Can you work these out from the model? Positions are in its coordinate system, mm. Round coordinates to 2 decimals unless told otherwise and drop trailing zeros. Write each loop counter-clockwise with the first axis right and the second up, starting at its lowest first coordinate (ties: lowest second). Pieces come first, ordered by that corner, then holes. Notation, with made-up numbers: M -1.75,51 L 41.25,51 A18 ccw 41.25,60 Z; hole C -38.75,69 d6. An arc over 180 degrees is marked long. Answer as a JSON object with one key per item and string values. Group by question number.
1) Suppose I cut it at C-C, the plane y = 22.5. Write out the boundary of the cut face in (x, z), and give its area (3 significant figures).
2) If we mould it in two halves opening along Z, with no side actions, what happens to faces 1 (the flat face through (-43, 25, 11)), 2 (the cylindrical face through (15.77, 12.325, 50.076)), 3 (the cylindrical face through (-42.954, 12.675, -9.538))? For each: +Z half, -Z half, draft (parallel to the pull), parting line (faces both ways), or undercut.
3) Suppose I cut it at B-B, the plane z = 0. Write out the boundary of the cut face in (x, y), and give its area (3 significant figures).
4) I'm going to push flat-ended pins straight in: pin 1 Ø6 at (x, y) = (-12, 16.5) entering from -Z; pin 2 Ø1.5 at (y, z) = (5.5, -37) entering from -X; pin 3 Ø4 at (y, z) = (19.5, -27) entering from +X. Where does each tip first touch, or does it pass through?
5) Suppose I cut it at A-A, the plane x = 0. Write out the boundary of the cut face in (y, z).
6) Please list where these lines run through material, in increasing order: L1, parallel to Z at x = 1, y = 4; L2, parallel to X at y = 16, z = 0; L3, parallel to Z at x = -27, y = 1 (3 decimals). Write a range as [from, to].
from build123d import *

# Parameters (mm, degrees)
SKETCH_1_R               = 52.5
SKETCH_1_R_2             = 11.15
EXTRUDE_1_DEPTH          = 25
CUT_EXTRUDE_1_DEPTH      = 30
PATTERN_CIRCULAR_1_COUNT = 6
FILLET_1_R               = 5
SKETCH_3_R               = 44
CUT_EXTRUDE_2_DEPTH      = 30


with BuildPart() as part:
    # 草图1 → 凸台-拉伸1 (new body)
    with BuildSketch(Plane(origin=(0, 0, 0), x_dir=(1, 0, 0), z_dir=(0, 1, 0))):
        with Locations(Location((0, 0, 0), (0, 0, 270))):
            Circle(SKETCH_1_R)
        with Locations(Location((0, 0, 0), (0, 0, 270))):
            Circle(SKETCH_1_R_2, mode=Mode.SUBTRACT)
    extrude(amount=EXTRUDE_1_DEPTH)

    # 草图2 → 切除-拉伸1 (cut)
    with BuildSketch(Plane(origin=(0, 25, 0), x_dir=(1, 0, 0), z_dir=(0, 1, 0))):
        with BuildLine():
            ThreePointArc((-21.398006208, 27.062433932), (-29.877876431, 17.25), (-34.135758377, 5))
            Line((-34.135758377, 5), (-21.15, 5))
            Line((-21.15, 5), (-20.550486612, 5))
            ThreePointArc((-20.550486612, 5), (-18.31643729, 10.575), (-14.605370325, 15.297243466))
            Line((-14.605370325, 15.297243466), (-14.905127019, 15.81643729))
            Line((-14.905127019, 15.81643729), (-21.398006208, 27.062433932))
        make_face()
    cut_extrude_1 = extrude(amount=-CUT_EXTRUDE_1_DEPTH, mode=Mode.SUBTRACT)

    # 阵列(圆周)1: 切除-拉伸1 ×6 about axis
    pattern_circular_1_axis = Axis((0, 25, 0), (0, -1, 0))
    for i in range(1, PATTERN_CIRCULAR_1_COUNT):
        add(cut_extrude_1.rotate(pattern_circular_1_axis, i * 360 / PATTERN_CIRCULAR_1_COUNT), mode=Mode.SUBTRACT)

    # 圆角1
    fillet_1_edges = [part.edges().sort_by_distance(p)[0] for p in [
        (-21.398006208, 12.5, -27.062433932),
        (-14.605370325, 12.5, -15.297243466),
        (-20.550486612, 12.5, -5),
        (-34.135758377, 12.5, -5),
        (-34.135758377, 12.5, 5),
        (-20.550486612, 12.5, 5),
        (-14.605370325, 12.5, 15.297243466),
        (-21.398006208, 12.5, 27.062433932),
        (-12.73775217, 12.5, 32.062433932),
        (-5.945116287, 12.5, 20.297243466),
        (5.945116287, 12.5, 20.297243466),
        (12.73775217, 12.5, 32.062433932),
        (21.398006208, 12.5, 27.062433932),
        (14.605370325, 12.5, 15.297243466),
        (20.550486612, 12.5, 5),
        (34.135758377, 12.5, 5),
        (34.135758377, 12.5, -5),
        (20.550486612, 12.5, -5),
        (14.605370325, 12.5, -15.297243466),
        (21.398006208, 12.5, -27.062433932),
        (12.73775217, 12.5, -32.062433932),
        (5.945116287, 12.5, -20.297243466),
        (-5.945116287, 12.5, -20.297243466),
        (-12.73775217, 12.5, -32.062433932),
    ]]
    fillet(fillet_1_edges, radius=FILLET_1_R)

    # 草图3 → 切除-拉伸2 (cut)
    with BuildSketch(Plane(origin=(0, 25, 0), x_dir=(1, 0, 0), z_dir=(0, 1, 0))):
        with Locations(Location((0, 0, 0), (0, 0, 270))):
            Circle(SKETCH_3_R)
        with BuildLine():
            ThreePointArc((9.546562067, -26.535130538), (9.751380834, -31.140900403), (6.100576582, -33.956339104))
            ThreePointArc((6.100576582, -33.956339104), (0, -34.5), (-6.100576582, -33.956339104))
            ThreePointArc((-6.100576582, -33.956339104), (-9.751380834, -31.140900403), (-9.546562067, -26.535130538))
            Line((-9.546562067, -26.535130538), (-7.751082565, -23.425268815))
            ThreePointArc((-7.751082565, -23.425268815), (-5.631733419, -21.440576943), (-2.766853147, -20.968238449))
            ThreePointArc((-2.766853147, -20.968238449), (0, -21.15), (2.766853147, -20.968238449))
            ThreePointArc((2.766853147, -20.968238449), (5.631733419, -21.440576943), (7.751082565, -23.425268815))
            Line((7.751082565, -23.425268815), (9.546562067, -26.535130538))
        make_face(mode=Mode.SUBTRACT)
        with BuildLine():
            ThreePointArc((27.753378173, -5), (31.844501263, -7.125506677), (32.457340575, -11.694915254))
            ThreePointArc((32.457340575, -11.694915254), (29.877876431, -17.25), (26.356763993, -22.26142385))
            ThreePointArc((26.356763993, -22.26142385), (22.093120428, -24.015393726), (18.206816105, -21.535130538))
            Line((18.206816105, -21.535130538), (16.411336602, -18.425268815))
            ThreePointArc((16.411336602, -18.425268815), (15.752217595, -15.59751268), (16.775600596, -12.880284338))
            ThreePointArc((16.775600596, -12.880284338), (18.31643729, -10.575), (19.542453743, -8.087954111))
            ThreePointArc((19.542453743, -8.087954111), (21.383951014, -5.843064263), (24.162419167, -5))
            Line((24.162419167, -5), (27.753378173, -5))
        make_face(mode=Mode.SUBTRACT)
        with BuildLine():
            ThreePointArc((-27.753378173, 5), (-31.844501263, 7.125506677), (-32.457340575, 11.694915254))
            ThreePointArc((-32.457340575, 11.694915254), (-29.877876431, 17.25), (-26.356763993, 22.26142385))
            ThreePointArc((-26.356763993, 22.26142385), (-22.093120428, 24.015393726), (-18.206816105, 21.535130538))
            Line((-18.206816105, 21.535130538), (-16.411336602, 18.425268815))
            ThreePointArc((-16.411336602, 18.425268815), (-15.752217595, 15.59751268), (-16.775600596, 12.880284338))
            ThreePointArc((-16.775600596, 12.880284338), (-18.31643729, 10.575), (-19.542453743, 8.087954111))
            ThreePointArc((-19.542453743, 8.087954111), (-21.383951014, 5.843064263), (-24.162419167, 5))
            Line((-24.162419167, 5), (-27.753378173, 5))
        make_face(mode=Mode.SUBTRACT)
        with BuildLine():
            ThreePointArc((-9.546562067, 26.535130538), (-9.751380834, 31.140900403), (-6.100576582, 33.956339104))
            ThreePointArc((-6.100576582, 33.956339104), (0, 34.5), (6.100576582, 33.956339104))
            ThreePointArc((6.100576582, 33.956339104), (9.751380834, 31.140900403), (9.546562067, 26.535130538))
            Line((9.546562067, 26.535130538), (7.751082565, 23.425268815))
            ThreePointArc((7.751082565, 23.425268815), (5.631733419, 21.440576943), (2.766853147, 20.968238449))
            ThreePointArc((2.766853147, 20.968238449), (0, 21.15), (-2.766853147, 20.968238449))
            ThreePointArc((-2.766853147, 20.968238449), (-5.631733419, 21.440576943), (-7.751082565, 23.425268815))
            Line((-7.751082565, 23.425268815), (-9.546562067, 26.535130538))
        make_face(mode=Mode.SUBTRACT)
        with BuildLine():
            ThreePointArc((18.206816105, 21.535130538), (22.093120428, 24.015393726), (26.356763993, 22.26142385))
            ThreePointArc((26.356763993, 22.26142385), (29.877876431, 17.25), (32.457340575, 11.694915254))
            ThreePointArc((32.457340575, 11.694915254), (31.844501263, 7.125506677), (27.753378173, 5))
            Line((27.753378173, 5), (24.162419167, 5))
            ThreePointArc((24.162419167, 5), (21.383951014, 5.843064263), (19.542453743, 8.087954111))
            ThreePointArc((19.542453743, 8.087954111), (18.31643729, 10.575), (16.775600596, 12.880284338))
            ThreePointArc((16.775600596, 12.880284338), (15.752217595, 15.59751268), (16.411336602, 18.425268815))
            Line((16.411336602, 18.425268815), (18.206816105, 21.535130538))
        make_face(mode=Mode.SUBTRACT)
    extrude(amount=-CUT_EXTRUDE_2_DEPTH, mode=Mode.SUBTRACT)


solid = part.part
Results:
{
 "1": {"outline": "C 0,0 d105; hole C 0,0 d88", "area": "2,580 mm^2"},
 "2": {"face 1": "draft", "face 2": "parting line", "face 3": "undercut"},
 "3": {"outline": "M -52.5,0 L -44,0 L -44,25 L -52.5,25 Z; M 44,0 L 52.5,0 L 52.5,25 L 44,25 Z", "area": "425 mm^2"},
 "4": {"pin 1": "z = -51.72", "pin 2": "x = -37.98", "pin 3": "x = 46.17"},
 "5": {"outline": "M 0,-52.5 L 25,-52.5 L 25,-44 L 0,-44 Z; M 0,44 L 25,44 L 25,52.5 L 0,52.5 Z"},
 "6": {"L1": "[-52.49, -43.99], [43.99, 52.49]", "L2": "[-52.5, -44], [44, 52.5]", "L3": "[-45.025, -34.742], [34.742, 45.025]"}
}
